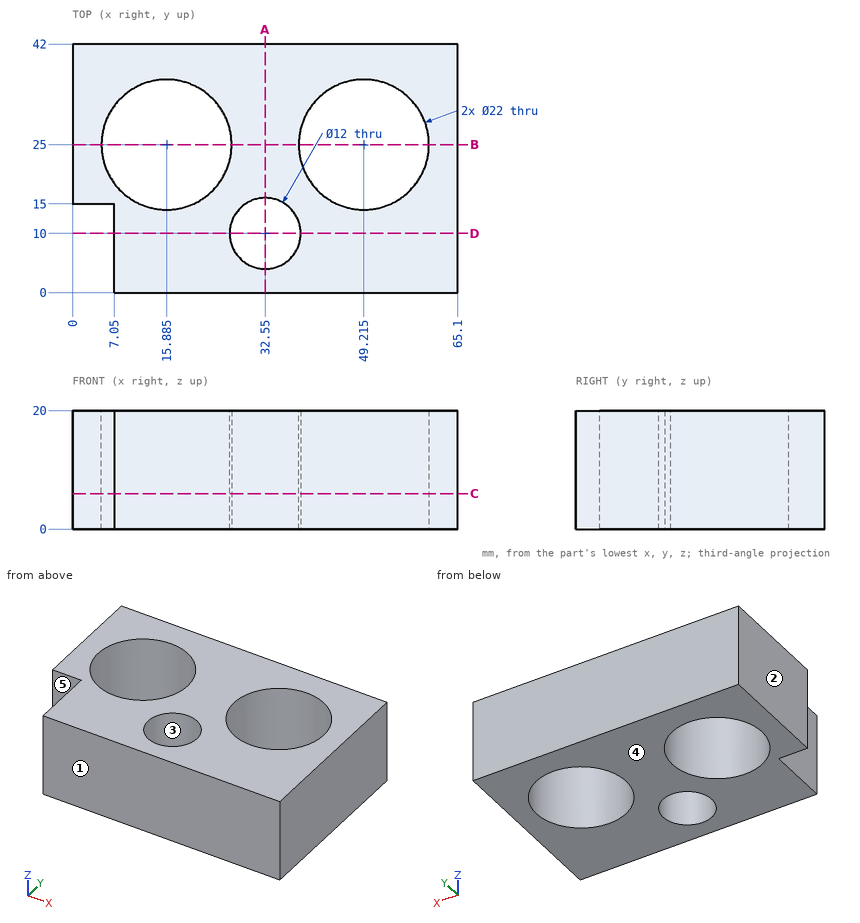
The drawing under review shows one solid part. Ordinate dimensions are in mm from its lowest x, y, z. A direction names the side the tool comes from. Round coordinates to 2 decimals unless told otherwise and drop trailing zeros. Order: outer loops, then holes, each group sorted by start corner. A loop starts at its lowest first (then second) coordinate and runs counter-clockwise, first axis right, second up. Notation, with made-up numbers: (-7.5, -19.5) -> (18.5, -19.5) arc R16 ccw to (18.5, -11.5) -> close; hole circle Ø9 at (84.25, 45). An arc over 180 degrees is marked (long way). Use a Markdown table: item, result.
Item 1: Take a section at B-B (y = 25). State the section outline as (x, z) points (3 decimals).
Resolved:
| item | result |
|---|---|
| outline | (0, 0) -> (4.885, 0) -> (4.885, 20) -> (0, 20) -> close; (26.885, 0) -> (38.215, 0) -> (38.215, 20) -> (26.885, 20) -> close; (60.215, 0) -> (65.1, 0) -> (65.1, 20) -> (60.215, 20) -> close |
Item 2: For line 1 along Y through (x, z) = (32.55, 15.75); line 2 along X through (y, z) = (33, 14.25); line 3 along Y through (x, z) = (49, 4.5), list the stretches that pass through material, from the lowest coordinate up. Write a range as [from, to].
Resolved:
| item | result |
|---|---|
| line 1 | y = [0, 4], [16, 42] |
| line 2 | x = [0, 8.34], [23.43, 41.67], [56.76, 65.1] |
| line 3 | y = [0, 14], [36, 42] |
Item 3: Draft analysis for pull direction Y (two halves, no side actions). For the marked faces 1, 2 and 3, state which applies: +Y half, -Y half, draft (parallel to the pull), parting line (faces both ways), or undercut.
Resolved:
| item | result |
|---|---|
| face 1 | -Y half |
| face 2 | draft |
| face 3 | undercut |
Item 4: Take a section at C-C (z = 6). State the section outline as (x, y) points (3 decimals), plus the area to 3 significant figures.
Resolved:
| item | result |
|---|---|
| outline | (0, 15) -> (7.05, 15) -> (7.05, 0) -> (65.1, 0) -> (65.1, 42) -> (0, 42) -> close; hole circle Ø22 at (15.885, 25); hole circle Ø12 at (32.55, 10); hole circle Ø22 at (49.215, 25) |
| area | 1,760 mm² |
Item 5: For pin 1 (1.5 mm diameter, centred on y = 8.5, z = 4, fed in from -X); pin 2 (8 mm diameter, centred on y = 15.5, z = 6.5, fed in from -X); pin 3 (3.5 mm diameter, centred on x = 3, z = 7, fed in from -Y), all flat-tipped, find the tip position at first contact; note any pin that passes through.
Resolved:
| item | result |
|---|---|
| pin 1 | stops at x = 7.05 |
| pin 2 | stops at x = 0 |
| pin 3 | stops at y = 15 |
Item 6: Take a section at D-D (y = 10). State the section outline as (x, z) points.
Resolved:
| item | result |
|---|---|
| outline | (7.05, 0) -> (26.55, 0) -> (26.55, 20) -> (7.05, 20) -> close; (38.55, 0) -> (65.1, 0) -> (65.1, 20) -> (38.55, 20) -> close |
Item 7: Machinability: for the marked faces 4 and 5, which of the approach directions +Z, -Z, +X, -X, +Y, -Y give a long, thin tool a straight path to every point of the face, cutting with its end or side? Answer none if there is none.
Resolved:
| item | result |
|---|---|
| face 4 | -Z, +X, -X, +Y, -Y |
| face 5 | +Z, -Z, -X, -Y |
Item 8: Take a section at A-A (x = 32.55). State the section outline as (y, z) points.
Resolved:
| item | result |
|---|---|
| outline | (0, 0) -> (4, 0) -> (4, 20) -> (0, 20) -> close; (16, 0) -> (42, 0) -> (42, 20) -> (16, 20) -> close |
